The listing builds one solid part. Answer for the finished solid, in the listing's coordinates (mm). Coordinates: 2 decimals unless noted, no trailing zeros. Write each loop counter-clockwise with the first axis right and the second up, starting at its lowest first coordinate (ties: lowest second). Pieces come first, ordered by that corner, then holes.
```python
from build123d import *

# Parameters (mm, degrees)
SKETCH1_R           = 1.75
SKETCH1_R_2         = 4.25
BOSS_EXTRUDE1_DEPTH = 6.35
FILLET1_R           = 5


with BuildPart() as part:
    # Sketch1 → Boss-Extrude1 (new body)
    with BuildSketch(Plane(origin=(0, 0, 0), x_dir=(1, 0, 0), z_dir=(0, 1, 0))):
        with BuildLine():
            Line((-5, 7.5), (29, 7.5))
            Line((29, 7.5), (29, -31.5))
            Line((29, -31.5), (19.150459769, -48.615024313))
            ThreePointArc((19.150459769, -48.615024313), (12, -52.75), (4.849540231, -48.615024313))
            Line((4.849540231, -48.615024313), (-5, -31.5))
            Line((-5, -31.5), (-5, 7.5))
        make_face()
        with Locations(Location((0, 0, 0), (0, 0, 270))):
            Circle(SKETCH1_R, mode=Mode.SUBTRACT)
        with Locations(Location((6, 0, 0), (0, 0, 270))):
            Circle(SKETCH1_R, mode=Mode.SUBTRACT)
        with Locations(Location((12, 0, 0), (0, 0, 270))):
            Circle(SKETCH1_R, mode=Mode.SUBTRACT)
        with Locations(Location((18, 0, 0), (0, 0, 270))):
            Circle(SKETCH1_R, mode=Mode.SUBTRACT)
        with Locations(Location((24, 0, 0), (0, 0, 270))):
            Circle(SKETCH1_R, mode=Mode.SUBTRACT)
        with Locations(Location((12, -44.5, 0), (0, 0, 270))):
            Circle(SKETCH1_R_2, mode=Mode.SUBTRACT)
    extrude(amount=BOSS_EXTRUDE1_DEPTH)

    # Fillet1
    fillet1_edges = [part.edges().sort_by_distance(p)[0] for p in [
        (29, 3.175, 31.5),
        (-5, 3.175, 31.5),
        (-5, 3.175, -7.5),
        (29, 3.175, -7.5),
    ]]
    fillet(fillet1_edges, radius=FILLET1_R)


solid = part.part
```
(1) Find the intervals of material crossed by probe 1 along X at (y, z) = (2.25, 0); probe 2 along Z at (x, y) = (15, 4); probe 3 along Z at (x, y) = (10.5, 3.25), in increasing order.
(2) Section C-C, the plane y = 5.5 is taken. Write down the section's boundary in (x, z), plus the area to 3 significant figures.
(3) Section D-D, the plane z = 44.5 is taken. Write down the section's boundary in (x, y).
(4) Section B-B, the plane z = 0 is taken. Write down the section's boundary in (x, y).
(5) For a pull along X with two mould halves and no side action, classify faces 1 (the flat face through (0.322, 3.131, 40.748)), 2 (the cylindrical face through (4.29, 3.13, -0.38)), 3 (the flat face through (23.81, 3.13, 40.52)) as pulls with the +X half, pulls with the -X half, needs draft (parallel to the pull), parting line crosses it, or undercut.
(6) Section A-A, the plane x = 12 is taken. Write down the section's boundary in (y, z), plus the area to 3 significant figures.
(7) This flat-tipped pin is pushed along its axis until it touches: pin 1 (2 mm diameter, centred on x = 0, z = 0, fed in from -Y). Where does it stop, or does it pass through?
Solution:
1. probe 1: x = -5 to -1.75, 1.75 to 4.25, 7.75 to 10.25, 13.75 to 16.25, 19.75 to 22.25, 25.75 to 29
1. probe 2: z = -7.5 to 41.49, 47.51 to 52.19
1. probe 3: z = -7.5 to -0.9, 0.9 to 40.52, 48.48 to 52.61
2. outline: (-5, -2.5) arc R5 ccw to (0, -7.5) - (24, -7.5) arc R5 ccw to (29, -2.5) - (29, 30.16) arc R5 ccw to (28.33, 32.66) - (19.15, 48.62) arc R8.25 ccw to (4.85, 48.62) - (-4.33, 32.66) arc R5 ccw to (-5, 30.16) - close; hole circle Ø3.5 at (0, 0); hole circle Ø3.5 at (6, 0); hole circle Ø8.5 at (12, 44.5); hole circle Ø3.5 at (12, 0); hole circle Ø3.5 at (18, 0); hole circle Ø3.5 at (24, 0)
2. area: 1,670 mm2
3. outline: (2.48, 0) - (7.75, 0) - (7.75, 6.35) - (2.48, 6.35) - close; (16.25, 0) - (21.52, 0) - (21.52, 6.35) - (16.25, 6.35) - close
4. outline: (-5, 0) - (-1.75, 0) - (-1.75, 6.35) - (-5, 6.35) - close; (1.75, 0) - (4.25, 0) - (4.25, 6.35) - (1.75, 6.35) - close; (7.75, 0) - (10.25, 0) - (10.25, 6.35) - (7.75, 6.35) - close; (13.75, 0) - (16.25, 0) - (16.25, 6.35) - (13.75, 6.35) - close; (19.75, 0) - (22.25, 0) - (22.25, 6.35) - (19.75, 6.35) - close; (25.75, 0) - (29, 0) - (29, 6.35) - (25.75, 6.35) - close
5. face 1: pulls with the -X half
5. face 2: undercut
5. face 3: pulls with the +X half
6. outline: (0, -7.5) - (6.35, -7.5) - (6.35, -1.75) - (0, -1.75) - close; (0, 1.75) - (6.35, 1.75) - (6.35, 40.25) - (0, 40.25) - close; (0, 48.75) - (6.35, 48.75) - (6.35, 52.75) - (0, 52.75) - close
6. area: 306 mm2
7. pin 1: passes through
